Autodesk Fusion 360 part; units mm, degrees
sketch "Sketch1" plane through (0, 0, 0) normal (0, 0, 1) x (1, 0, 0)
  line L0 (0, 0) -> (79, 0)
  line L1 (79, 0) -> (79, 44)
  line L2 (79, 44) -> (0, 44)
  line L3 (0, 44) -> (0, 0)
  circle A0 centre (5, 39) radius 1.7
  circle A1 centre (5, 39) radius 3.7
  circle A2 centre (74, 5) radius 1.7
  circle A3 centre (74, 5) radius 3.7
  line L4 (1.2, 42.8) -> (77.8, 42.8)
  line L5 (77.8, 42.8) -> (77.8, 1.2)
  line L6 (77.8, 1.2) -> (1.2, 1.2)
  line L7 (1.2, 1.2) -> (1.2, 42.8)
  dimension "d1" = 44
  dimension "d2" = 79
  dimension "d30" = 3.4
  dimension "d31" = 7.4
  dimension "d34" = 3.4
  dimension "d35" = 7.4
  dimension "d46" = 1.2
  dimension "d47" = 1.2
  dimension "d48" = 1.2
  dimension "d49" = 1.2
  dimension "d50" = 3.8
  dimension "d51" = 3.8
  dimension "d52" = 3.8
  dimension "d53" = 3.8
extrude "Extrude5" add sketch "Sketch1" along normal blind 11 contours A1 | A3 makes body 1 at (8.6954, 38.8156, 7.3333) makes body 2 at (77.6954, 4.8156, 7.3333)
extrude "Extrude6" add sketch "Sketch1" along normal blind 9 contours L0 L1 L2 L3 | L4 L5 L6 L7 bodies 1 2
extrude "Extrude7" cut sketch "Sketch1" along normal blind 2.6 contours A1 bodies 1
extrude "Extrude8" cut sketch "Sketch1" along normal blind 2.6 contours A0 | A1 | A3 bodies 1
Build history of the part. All positions in model axes, mm. A direction names the side the tool comes from. Give positions to 0.01 mm unless a question says otherwise; leave off trailing zeros. Loops run counter-clockwise (first coordinate to the right, second up) from the corner with the lowest first, then second, coordinate; pieces in that order, holes last. Notation, with made-up numbers: (20, 17) -> (73, 17) arc R7 cw to (73, 22) -> close; hole circle Ø6 at (-34.75, 38.5). An arc over 180 degrees is marked (long way). Answer in a Markdown table with one row per item.
Item 1: Slice it at D-D on z = 1.75. Write the cut outline in (x, y).
Findings below:
| item | result |
|---|---|
| outline | (0, 0) -> (79, 0) -> (79, 44) -> (0, 44) -> close; hole circle Ø7.4 at (5, 39); hole circle Ø7.4 at (74, 5) |
Item 2: Mould opens along X. For faces 1 (the cylindrical face through (70.304, 4.837, 1.282)), 2 (the flat face through (79, 22, 4)), 3 (the flat face through (76, 4, 11)) say: pulls with the +X half, pulls with the -X half, needs draft (parallel to the pull), parting line crosses it, or undercut.
Findings below:
| item | result |
|---|---|
| face 1 | undercut |
| face 2 | pulls with the +X half |
| face 3 | needs draft |
Item 3: Slice it at B-B on z = 9.75. Write the cut outline in (x, y).
Findings below:
| item | result |
|---|---|
| outline | circle Ø7.4 at (5, 39); circle Ø7.4 at (74, 5); hole circle Ø3.4 at (5, 39); hole circle Ø3.4 at (74, 5) |
Item 4: Tool access for faces 4 (the cylindrical face through (4.52, 35.33, 9.99)), 5 (the flat face through (6, 37, 2.6)), 6 (the cylindrical face through (4.63, 40.66, 6.74)): list every direction of +Z, -Z, +X, -X, +Y, -Y with a clear straight run to the whole face (end or side of a thin tool).
Findings below:
| item | result |
|---|---|
| face 4 | +Z |
| face 5 | -Z |
| face 6 | +Z, -Z |
Item 5: Flat gauge pins, fed straight in: P1, Ø5.5, axis at x = 74, y = 5, coming from the -Z side; P2, Ø2, axis at x = 11, y = 25.5, coming from the +Z side. Where does each tip first touch, or does it go through?
Findings below:
| item | result |
|---|---|
| P1 | stops at z = 2.6 |
| P2 | stops at z = 9 |
Item 6: Probe line 1 along Y through (x, z) = (5, 1.25); line 2 along Y through (x, z) = (5, 6); line 3 along Z through (x, y) = (66.5, 15). List the from-to ranges inside material, lowest first. Write a range as [from, to].
Findings below:
| item | result |
|---|---|
| line 1 | y = [0, 35.3], [42.7, 44] |
| line 2 | y = [0, 37.3], [40.7, 44] |
| line 3 | z = [0, 9] |
Item 7: Slice it at C-C on y = 5. Write the cut outline in (x, z).
Findings below:
| item | result |
|---|---|
| outline | (0, 0) -> (70.3, 0) -> (70.3, 2.6) -> (72.3, 2.6) -> (72.3, 11) -> (70.3, 11) -> (70.3, 9) -> (0, 9) -> close; (75.7, 2.6) -> (77.7, 2.6) -> (77.7, 0) -> (79, 0) -> (79, 9) -> (77.7, 9) -> (77.7, 11) -> (75.7, 11) -> close |
Item 8: Slice it at A-A on x = 5. Write the cut outline in (y, z), plus the area to 3 significant figures.
Findings below:
| item | result |
|---|---|
| outline | (0, 0) -> (35.3, 0) -> (35.3, 2.6) -> (37.3, 2.6) -> (37.3, 11) -> (35.3, 11) -> (35.3, 9) -> (0, 9) -> close; (40.7, 2.6) -> (42.7, 2.6) -> (42.7, 0) -> (44, 0) -> (44, 9) -> (42.7, 9) -> (42.7, 11) -> (40.7, 11) -> close |
| area | 363 mm² |
